Could you check a few things on this model? Use its own coordinates, in mm. Coordinates: 2 decimals unless noted, no trailing zeros. Write each loop counter-clockwise with the first axis right and the second up, starting at its lowest first coordinate (ties: lowest second). Pieces come first, ordered by that corner, then holes.
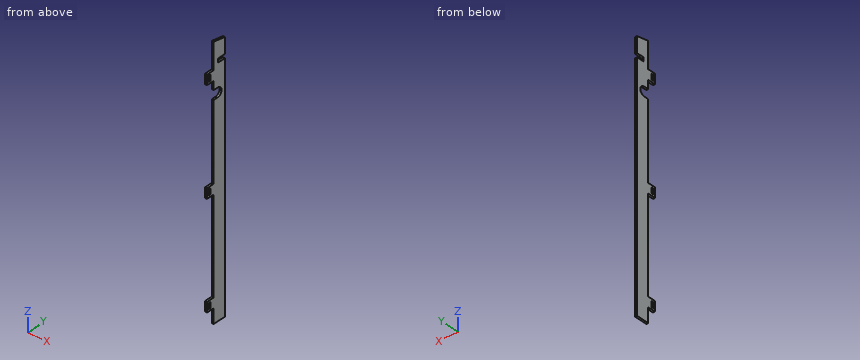
Autodesk Inventor part; units mm, degrees
ref_plane "YZ Plane" through (0, 0, 0) normal (1, 0, 0) x (0, 1, 0)
ref_plane "XZ Plane" through (0, 0, 0) normal (0, 1, 0) x (-1, 0, 0)
ref_plane "XY Plane" through (0, 0, 0) normal (0, 0, 1) x (1, 0, 0)
sketch "Sketch2" plane through (0, 0, 0) normal (0, 1, 0) x (-1, 0, 0)
  line L0 (-1.5, -198.6195) -> (1.5, -198.6195)
  line L1 (1.5, -198.6195) -> (1.5, 198.6195)
  line L2 (1.5, 198.6195) -> (-1.5, 198.6195)
  line L3 (-1.5, 198.6195) -> (-1.5, -198.6195)
  line L4 (-1.5, -198.6195) -> (1.5, 198.6195) construction
  line L5 (1.5, -198.6195) -> (-1.5, 198.6195) construction
  point P0 (0, 0)
  dimension "d0" = 3
  dimension "d1" = 397.239
extrude "Extrusion1" add sketch "Sketch2" along normal blind 20
sketch "Sketch3" plane through (1.5, 0, 198.6195) normal (1, 0, 0) x (0, 0, -1)
  line L0 (397.239, 0) -> (0, 0)
  line L1 (68, 0) -> (82, 0)
  line L2 (82, 0) -> (82, 7)
  line L3 (68, 7) -> (68, 0)
  arc A0 (82, 7) -> (68, 7) centre (75, 7) ccw
  arc A1 (68, 7) -> (82, 7) centre (75, 7) ccw construction
  line L4 (0, 0) -> (0, 20)
  point P0 (198.6195, 0)
  dimension "d4" = 14
  dimension "d5" = 7
  dimension "d6" = 14
  dimension "d9" = 75
extrude "Extrusion2" cut sketch "Sketch3" against normal through all
sketch "Sketch4" plane through (1.5, 0, -198.6195) normal (1, 0, 0) x (0, 0, -1)
  line L0 (-329.239, 0) -> (-397.239, 0)
  line L1 (-397.239, 0) -> (-397.239, 20)
  line L2 (-397.239, 0) -> (-397.239, 20)
  line L3 (-397.239, 20) -> (-393.7125, 20)
  line L4 (-397.239, 20) -> (0, 20)
  line L5 (-397.239, 0) -> (-393.7125, 20)
  point P0 (-198.6195, 0)
  dimension "d10" = 10
extrude "Extrusion3" cut sketch "Sketch4" against normal through all
sketch "Sketch6" plane through (1.5, 0, -198.6195) normal (1, 0, 0) x (0, 0, -1)
  line L0 (-393.7125, 20) -> (0, 20)
  line L1 (-369.839, 20) -> (-363.839, 20)
  line L2 (-363.839, 20) -> (-363.839, 8)
  line L3 (-363.839, 8) -> (-369.839, 8)
  line L4 (-369.839, 8) -> (-369.839, 20)
  line L5 (-329.239, 0) -> (-397.239, 0) construction
  line L6 (-397.239, 0) -> (-397.239, 30) construction
  point P0 (-198.6195, 0)
  dimension "d20" = 6
  dimension "d21" = 12
  dimension "d25" = 27.4
extrude "Extrusion5" cut sketch "Sketch6" against normal blind 6
sketch "Sketch7" plane through (1.5, 0, -198.6195) normal (1, 0, 0) x (0, 0, -1)
  line L0 (-357.239, 0) -> (-342.239, 0)
  line L1 (-342.239, 0) -> (-342.239, -12)
  line L2 (-342.239, -12) -> (-357.239, -12)
  line L3 (-357.239, -12) -> (-357.239, 0)
  line L4 (-354.239, -6) -> (-345.239, -6)
  line L5 (-345.239, -6) -> (-345.239, -9)
  line L6 (-345.239, -9) -> (-354.239, -9)
  line L7 (-354.239, -9) -> (-354.239, -6)
  line L8 (-397.239, 0) -> (-329.239, 0)
  line L9 (-197.239, 0) -> (-182.239, 0)
  line L10 (-182.239, 0) -> (-182.239, -12)
  line L11 (-182.239, -12) -> (-197.239, -12)
  line L12 (-197.239, -12) -> (-197.239, 0)
  line L13 (-194.239, -6) -> (-185.239, -6)
  line L14 (-185.239, -6) -> (-185.239, -9)
  line L15 (-185.239, -9) -> (-194.239, -9)
  line L16 (-194.239, -9) -> (-194.239, -6)
  line L17 (-37.239, 0) -> (-22.239, 0)
  line L18 (-22.239, 0) -> (-22.239, -12)
  line L19 (-22.239, -12) -> (-37.239, -12)
  line L20 (-37.239, -12) -> (-37.239, 0)
  line L21 (-34.239, -6) -> (-25.239, -6)
  line L22 (-25.239, -6) -> (-25.239, -9)
  line L23 (-25.239, -9) -> (-34.239, -9)
  line L24 (-34.239, -9) -> (-34.239, -6)
  line L25 (-315.239, 0) -> (0, 0)
  point P0 (-198.6195, 0)
  dimension "d26" = 15
  dimension "d27" = 3
  dimension "d28" = 6
  dimension "d29" = 3
  dimension "d30" = 3
  dimension "d31" = 3
  dimension "d32" = 40
  dimension "d33" = 15
  dimension "d34" = 3
  dimension "d35" = 6
  dimension "d36" = 3
  dimension "d37" = 3
  dimension "d38" = 3
  dimension "d39" = 15
  dimension "d40" = 3
  dimension "d41" = 6
  dimension "d42" = 3
  dimension "d43" = 3
  dimension "d44" = 3
  dimension "d45" = 145
  dimension "d46" = 145
extrude "Extrusion6" add sketch "Sketch7" against normal blind 3
equation "\"d30\" = d29"
equation "\"d31\" = d29"
equation "\"d37\" = d36"
equation "\"d38\" = d36"
equation "\"d43\" = d42"
equation "\"d44\" = d42"
properties part number "wall-inner-plunger"
1. I want a section at B-B on z = -105. Please give me the cut outline in (x, y).
Verdict:
outline: (-1.5, 0) - (1.5, 0) - (1.5, 20) - (-1.5, 20) - close
2. Please list where these lines run through material, in increasing order: line 1 along Z through (x, y) = (0.65, -2); line 2 along Y through (x, z) = (-0.75, -9); line 3 along Z through (x, y) = (-0.25, 9).
Verdict:
line 1: z = -176.38 to -161.38, -16.38 to -1.38, 143.62 to 158.62
line 2: y = -12 to -9, -6 to 20
line 3: z = -198.62 to 116.91, 130.33 to 165.22, 171.22 to 197.03
3. For pin 1 (1.5 mm diameter, centred on x = 0, z = 109, fed in from -Y); pin 2 (0.9 mm diameter, centred on x = 0.5, y = -7, fed in from -Z), each with a flat end and sliding along its axis, tell me the tip position at first contact or that it passes through.
Verdict:
pin 1: stops at y = 0
pin 2: stops at z = -176.38
4. I want a section at A-A on x = 0. Give the number of separate pieces and of enclosed holes in the cut face, plus the area to 3 significant figures.
Verdict:
separate pieces: 1
enclosed holes: 3
area: 8,120 mm2
